Model file for the job. Use its own axes, mm. A direction names the side the tool comes from. Round coordinates to 2 decimals unless told otherwise and drop trailing zeros. Order: outer loops, then holes, each group sorted by start corner. A loop starts at its lowest first (then second) coordinate and runs counter-clockwise, first axis right, second up. Notation, with made-up numbers: (-30.5, 51) - (-18.5, 51) arc R25 cw to (-18.5, 74) - close; hole circle Ø7 at (46.5, 26). An arc over 180 degrees is marked (long way). Answer as CSV lines item,"result". Start each with the question number.
1. 3-axis set-ups, long thin cutter, end or side, ignore diameter. For faces 4 (the face through (-7.395, -15.022, 19.468)), 5 (the face through (17, 10, -1)), 6 (the face through (0, -7, -49)): which of +Z, -Z, +X, -X, +Y, -Y reach the whole face in a straight line?
2. Band-saw the part on D-D on y = -2. List the corners of the cut face in (x, z), then the cut area to 3 significant figures.
3. Wall check: line 1 along Y through (x, z) = (12, -11); line 2 along X through (y, z) = (-20, 22.5); line 3 along Z through (x, y) = (29, 4.5). Give the ranges that are in metal, low to high. Write a range as [from, to].
4. Pull direction Y, two halves, no side cores. Call faces 1 (the face through (-7.395, -15.448, -13.306)), 2 (the face through (48.61, 0.14, 4.91)), 3 (the face through (0, 0, 32)): released by +Y, released by -Y, zero draft, split by the parting line, or undercut.
5. Pin check, flat tips, straight feed: pin 1 Ø3 at (x, z) = (46.5, -4.5) entering from +Y; pin 2 Ø18.5 at (y, z) = (20, -11.5) entering from +X; pin 3 Ø10 at (y, z) = (1.5, 37) entering from -X. Stop position of each tip, or through.
6. Band-saw the part on A-A on z = 26. List the corners of the cut face in (x, y).
7. Band-saw the part on B-B on x = -4. List the corners of the cut face in (y, z), then the cut area to 3 significant figures.
8. Band-saw the part on C-C on z = 12. List the corners of the cut face in (x, y), then the cut area to 3 significant figures.
```python
from build123d import *

# Parameters (mm, degrees)
F2_DEPTH      = 15
F3_DEPTH      = 10
F3_DEPTH_BACK = 10


# Not quite as in the source:
# - a feature names something its author has since deleted; it is built from what else it names


with BuildPart() as f2:
    # F1 (on Right) → F2 (new body)
    with BuildSketch(Plane.YZ):
        Polygon((32.8475944698, 30.4612312466), (0, 9.1243321076), (-30.4703023285, 30.1044266671), (0, -57.9494014382), align=None)
    extrude(amount=-F2_DEPTH)

    # F0 (on Front) → F3 (join, two sides)
    with BuildSketch(Plane.XZ) as f3_sk:
        Polygon((35.6550849974, 0), (0, 53.336199373), (0, -57.4131049216), (61.2032115459, 9.6858292818), align=None)
    extrude(amount=-F3_DEPTH)
    extrude(f3_sk.sketch, amount=F3_DEPTH_BACK)


solid = f2.part
```
Reply:
1,face 4,"+Z, -X"
1,face 5,"+Z, -Z, +X, +Y"
1,face 6,"-Z, -X, -Y"
2,outline,"(-15, -52.17) - (0, -52.17) - (0, -57.41) - (61.2, 9.69) - (35.66, 0) - (0, 53.34) - (0, 10.5) - (-15, 10.5) - close"
2,area,"3,480 mm2"
3,line 1,"y = [-10, 10]"
3,line 2,"x = [-15, 0]"
3,line 3,"z = [-25.62, 9.96]"
4,face 1,"released by -Y"
4,face 2,"zero draft"
4,face 3,"undercut"
5,pin 1,"stops at y = 10"
5,pin 2,"stops at x = 0"
5,pin 3,"stops at x = 0"
6,outline,"(-15, -29.05) - (0, -29.05) - (0, -24.51) - (-15, -24.51) - close; (-15, 25.98) - (0, 25.98) - (0, 31.19) - (-15, 31.19) - close; (0, -10) - (18.27, -10) - (18.27, 10) - (0, 10) - close"
7,outline,"(-30.47, 30.1) - (0, -57.95) - (32.85, 30.46) - (0, 9.12) - close"
7,area,"2,120 mm2"
8,outline,"(-15, -24.21) - (0, -24.21) - (0, -10) - (27.63, -10) - (27.63, 10) - (0, 10) - (0, 25.99) - (-15, 25.99) - (-15, 4.43) - (0, 4.43) - (0, -4.18) - (-15, -4.18) - close"
8,area,"1,180 mm2"
